Part print with two shaded views. Sizes in mm from the minimum x, y, z corner. A direction names the side the tool comes from. Round coordinates to 2 decimals unless told otherwise and drop trailing zeros. Loops run counter-clockwise (first coordinate to the right, second up) from the corner with the lowest first, then second, coordinate; pieces in that order, holes last. Notation, with made-up numbers: M -31,2 L 6,2 A21 cw 6,32 Z; hole C 49.25,39.5 d10. An arc over 180 degrees is marked long. Use a Markdown table: item, result. Add a question column.
Item 1: Saw through at A-A on x = 3.1. Write the cut outline in (y, z), then the cut area to 3 significant figures.
Item 2: Tool access for the marked faces 1 and 2: list every direction of +Z, -Z, +X, -X, +Y, -Y with a clear straight run to the whole face (end or side of a thin tool).
Item 3: Saw through at D-D on z = 5.25. Write the cut outline in (x, y), then the cut area to 3 significant figures.
Item 4: Wall check: L1, parallel to Z at x = 3.1, y = 3; L2, parallel to Z at x = 3.1, y = 7. Give the ranges that are in metal, low to high. Write a range as from..to.
Item 5: Saw through at C-C on y = 9. Write the cut outline in (x, z), then the cut area to 3 significant figures.
Item 6: Saw through at B-B on z = 3.1. Write the cut outline in (x, y), then the cut area to 3 significant figures.
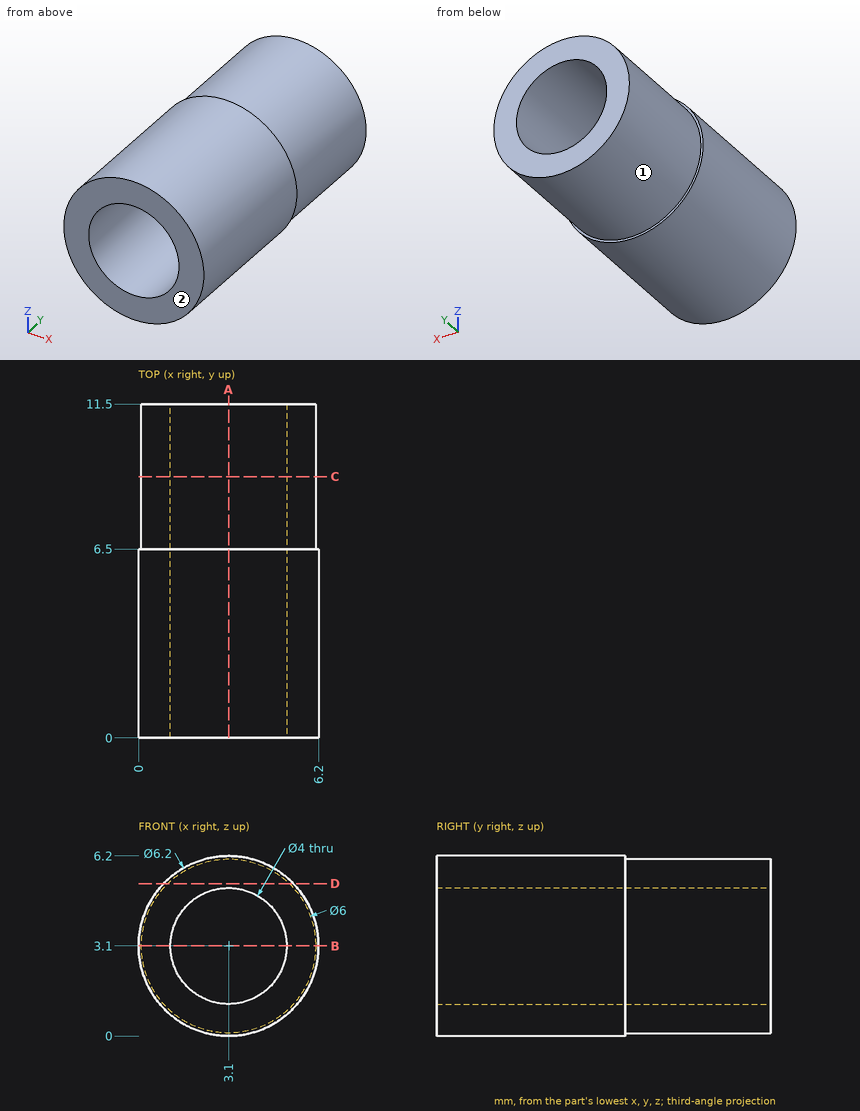
Entries:
| question | item | result |
|---|---|---|
| 1 | outline | M 0,0 L 6.5,0 L 6.5,0.1 L 11.5,0.1 L 11.5,1.1 L 0,1.1 Z; M 0,5.1 L 11.5,5.1 L 11.5,6.1 L 6.5,6.1 L 6.5,6.2 L 0,6.2 Z |
| 1 | area | 24.3 mm2 |
| 2 | face 1 | +Y |
| 2 | face 2 | +Z, -Z, +X, -X, -Y |
| 3 | outline | M 0.87,0 L 5.33,0 L 5.33,6.5 L 5.19,6.5 L 5.19,11.5 L 1.01,11.5 L 1.01,6.5 L 0.87,6.5 Z |
| 3 | area | 50.0 mm2 |
| 4 | L1 | 0..1.1, 5.1..6.2 |
| 4 | L2 | 0.1..1.1, 5.1..6.1 |
| 5 | outline | C 3.1,3.1 d6; hole C 3.1,3.1 d4 |
| 5 | area | 15.7 mm2 |
| 6 | outline | M 0,0 L 1.1,0 L 1.1,11.5 L 0.1,11.5 L 0.1,6.5 L 0,6.5 Z; M 5.1,0 L 6.2,0 L 6.2,6.5 L 6.1,6.5 L 6.1,11.5 L 5.1,11.5 Z |
| 6 | area | 24.3 mm2 |
